Input: part model. Units: mm. Frame: model coordinates. A direction names the side the tool comes from. Coordinates: 2 decimals unless noted, no trailing zeros. Order: outer loops, then holes, each group sorted by start corner. A loop starts at its lowest first (then second) coordinate and runs counter-clockwise, first axis right, second up.
from build123d import *

# Parameters (mm, degrees)
F0_W          = 174.6804863214
F0_H          = 6.394301774
F1_DEPTH      = 67.056
F2_ANGLE      = 10
F3_W          = 174.6804863214
F3_H          = 6.0367527984
F3_H_2        = 3.3486538234
F3_H_3        = 4.6590082347
F3_H_4        = 3.4464076161
F3_H_5        = 3.4266933799
F3_H_6        = 3.1117796898
F4_DEPTH      = 0.635
F5_DEPTH      = 32.766
F5_DEPTH_BACK = 6.35
F6_R          = 5.08
F7_W          = 5.0366173964
F7_H          = 42.1194909459
F7_W_2        = 179.0462706704
F8_DEPTH      = 2.032


with BuildPart() as f1:
    # F0 (on Front) → F1 (new body)
    with BuildSketch(Plane.XZ):
        with Locations((4.4365723152, 0.0675924821)):
            Rectangle(F0_W, F0_H)
    extrude(amount=F1_DEPTH)


with BuildPart() as f1_1:
    # F2: moved
    add(f1.part.rotate(Axis((4.4365723152, 0, 3.2647433691), (1, 0, 0)), F2_ANGLE))

    # F3 (on face) → F4 (join)
    with BuildSketch(Plane(origin=(0, -0.5583039975, 3.1662993109), x_dir=(1, 0, 0), z_dir=(0, -0.1736481777, 0.984807753))):
        with Locations((4.4365723152, -17.1857467104)):
            Rectangle(F3_W, F3_H)
        with Locations((4.4365723152, -31.2867563517)):
            Rectangle(F3_W, F3_H_2)
        with Locations((4.4365723152, -27.2829253227)):
            Rectangle(F3_W, F3_H_3)
        with Locations((4.4365723152, -46.3344976306)):
            Rectangle(F3_W, F3_H_4)
        with Locations((4.4365723152, -55.3813166916)):
            Rectangle(F3_W, F3_H_5)
        with Locations((4.4365723152, -63.4787082672)):
            Rectangle(F3_W, F3_H_6)
    extrude(amount=F4_DEPTH)

    # F3 (on face) → F5 (join, two sides)
    with BuildSketch(Plane(origin=(0, -0.5583039975, 3.1662993109), x_dir=(1, 0, 0), z_dir=(0, -0.1736481777, 0.984807753))) as f5_sk:
        Polygon((-82.9036708456, -66.4890832634), (-82.9036708456, -65.0345981121), (-82.9036708456, -61.9228184223), (-82.9036708456, -57.0946633816), (-82.9036708456, -53.6679700017), (-82.9036708456, -48.0577014387), (-82.9036708456, -44.6112938225), (-82.9036708456, -36.0245257616), (-82.9036708456, -32.9610832634), (-82.9036708456, -29.61242944), (-82.9036708456, -24.9534212053), (-82.9036708456, -20.2041231096), (-82.9036708456, -14.1673703112), (-87.36910671, -14.1673703112), (-87.36910671, -66.4890832634), align=None)
        Polygon((91.7768154759, -61.9228184223), (91.7768154759, -65.0345981121), (91.7768154759, -66.4890832634), (96.8134328723, -66.4890832634), (96.8134328723, -14.1673703112), (91.7768154759, -14.1673703112), (91.7768154759, -20.2041231096), (91.7768154759, -24.9534212053), (91.7768154759, -29.61242944), (91.7768154759, -32.9610832634), (91.7768154759, -36.0245257616), (91.7768154759, -44.6112938225), (91.7768154759, -48.0577014387), (91.7768154759, -53.6679700017), (91.7768154759, -57.0946633816), align=None)
    extrude(amount=F5_DEPTH)
    extrude(f5_sk.sketch, amount=-F5_DEPTH_BACK)

    # F6
    f6_edges = [f1_1.edges().sort_by_distance(p)[0] for p in [
        (94.295124, -20.200196, 32.974372),
        (-85.136389, -20.200196, 32.974372),
        (-85.136389, -71.727025, 23.888802),
        (94.295124, -71.727025, 23.888802),
    ]]
    fillet(f6_edges, radius=F6_R)

    # F7 (on face) → F8 (join)
    with BuildSketch(Plane(origin=(0, -6.2480601869, 35.4345101461), x_dir=(1, 0, 0), z_dir=(0, -0.1736481777, 0.984807753))):
        with Locations((94.2951241741, -40.3493377905)):
            Rectangle(F7_W, F7_H)
        with Locations((2.2536801407, -40.3493377905)):
            Rectangle(F7_W_2, F7_H)
    extrude(amount=F8_DEPTH)


solid = f1_1.part
Item 1: Access query for faces 5 (the face through (3.214, -17.552, 0.815)), 6 (the face through (3.214, -7.154, 2.003)). Directions: +Z, -Z, +X, -X, +Y, -Y. A direction counts if a zero-diameter tool reaches every point of the face in a straight line with its end or side. Return the directions, or none.
Response values:
face 5: +Z, -Y
face 6: +Z, +X, -X
Item 2: Cut plane B-B on z = 9.5. Return loops of the section in (x, y).
Response values:
outline: (-87.37, -69.19) - (-82.9, -69.19) - (-82.9, -16.06) - (-87.37, -16.06) - close; (91.78, -69.19) - (96.81, -69.19) - (96.81, -16.06) - (91.78, -16.06) - close
Item 3: Cut plane D-D on z = -10.5. Return loops of the section in (x, y).
Response values:
outline: (-87.37, -65.66) - (96.81, -65.66) - (96.81, -41.5) - (91.78, -41.5) - (91.78, -41.24) - (-82.9, -41.24) - (-82.9, -41.5) - (-87.37, -41.5) - close
Item 4: Pin query (flat end, axial travel): pin 1 Ø12 at (x, y) = (36.5, -8) entering from +Z; pin 2 Ø3 at (y, z) = (-17.5, -7.5) entering from +X; pin 3 Ø5 at (x, y) = (-38.5, -36) entering from -Z; pin 4 Ø6 at (x, y) = (26.5, -44.5) entering from -Z. Return the tip coordinate at first contact, or that it passes through.
Response values:
pin 1: stops at z = 2.91
pin 2: stops at x = 96.81
pin 3: stops at z = -10.02
pin 4: stops at z = -11.6
Item 5: Cut plane A-A on x = 51.5. Return loops of the section in (y, z), then the cut area to 3 significant figures.
Response values:
outline: (-67.08, 26.77) - (-66.72, 24.77) - (-25.24, 32.08) - (-25.6, 34.09) - close; (-66.04, -8.38) - (-64.93, -14.68) - (1.11, -3.03) - (0, 3.26) - (-14.51, 0.71) - (-14.62, 1.33) - (-20.57, 0.28) - (-20.46, -0.34) - (-25.13, -1.17) - (-25.24, -0.54) - (-33.13, -1.93) - (-33.02, -2.56) - (-44.49, -4.58) - (-44.6, -3.96) - (-48, -4.55) - (-47.89, -5.18) - (-53.41, -6.15) - (-53.52, -5.53) - (-56.9, -6.12) - (-56.79, -6.75) - (-61.54, -7.59) - (-61.65, -6.96) - (-64.72, -7.5) - (-64.6, -8.13) - close
area: 530 mm2
Item 6: Draft query along X for faces 1 (the face through (3.21, -59.13, -7.16)), 2 (the face through (-82.904, -8, -2)), 3 (the face through (3.214, -63.161, -7.228)), 4 (the face through (91.777, -8, -2)). Return one class per face: pulls with the +X half, pulls with the -X half, needs draft (parallel to the pull), parting line crosses it, or undercut.
Response values:
face 1: undercut
face 2: pulls with the -X half
face 3: undercut
face 4: pulls with the +X half
Item 7: Cut plane C-C on y = -41. Return loops of the section in (x, z).
Response values:
outline: (-87.37, -10.41) - (-82.9, -10.41) - (-82.9, -10.46) - (91.78, -10.46) - (91.78, -10.41) - (96.81, -10.41) - (96.81, 31.37) - (-87.27, 31.37) - (-87.27, 29.31) - (-87.37, 29.31) - close; hole (-82.9, -3.96) - (91.78, -3.96) - (91.78, 29.31) - (-82.9, 29.31) - close
Item 8: Ray query, probe 1 along X at (y, z) = (-22.5, 11); probe 2 along Z at (x, y) = (38.5, -57.5); probe 3 along Z at (x, y) = (-69, -41). Return the intervals inside material, ascending.
Response values:
probe 1: x = -87.37 to -82.9, 91.78 to 96.81
probe 2: z = -13.37 to -6.87, 26.4 to 28.46
probe 3: z = -10.46 to -3.96, 29.31 to 31.37
